from build123d import *
from build123d.topology import SkipClean

# Parameters (mm, degrees)
BOSS_EXTRUDE1_DEPTH   = 25
BOSS_EXTRUDE1_2_DEPTH = 25
BOSS_EXTRUDE1_3_DEPTH = 25
BOSS_EXTRUDE1_4_DEPTH = 25
BOSS_EXTRUDE1_5_DEPTH = 25
BOSS_EXTRUDE1_6_DEPTH = 25
BOSS_EXTRUDE1_7_DEPTH = 25
BOSS_EXTRUDE1_8_DEPTH = 25
BOSS_EXTRUDE2_START   = -3
SKETCH6_R             = 33
SKETCH6_R_2           = 31.685
BOSS_EXTRUDE2_DEPTH   = 3


with BuildPart() as part:
    # Sketch1 → Boss-Extrude1 (new body)
    with BuildSketch(Plane(origin=(0, 0, 0), x_dir=(-1, 0, 0), z_dir=(0, 0, 1))):
        with BuildLine():
            Line((-1.738225696, 20.20466707), (-2.272785403, 26.41824505))
            ThreePointArc((-2.272785403, 26.41824505), (-3.462351882, 28.561557475), (-5.853284272, 29.102204182))
            ThreePointArc((-5.853284272, 29.102204182), (-11.35995769, 27.425363923), (-16.439468924, 24.717262925))
            ThreePointArc((-16.439468924, 24.717262925), (-17.747818477, 22.644323466), (-17.073418251, 20.287622193))
            Line((-17.073418251, 20.287622193), (-13.05774592, 15.515968274))
            ThreePointArc((-13.05774592, 15.515968274), (-11.238150281, 14.485616628), (-9.187418979, 14.894338942))
            ThreePointArc((-9.187418979, 14.894338942), (-6.696960066, 16.167891819), (-4.035401805, 17.028374328))
            ThreePointArc((-4.035401805, 17.028374328), (-2.296305475, 18.189450019), (-1.738225696, 20.20466707))
        make_face()
    extrude(amount=BOSS_EXTRUDE1_DEPTH)



with BuildPart() as body_2:
    # Sketch1 → Boss-Extrude1 2 (new body)
    with BuildSketch(Plane(origin=(0, 0, 0), x_dir=(-1, 0, 0), z_dir=(0, 0, 1))):
        with BuildLine():
            Line((1.738225696, 20.20466707), (2.272785403, 26.41824505))
            ThreePointArc((2.272785403, 26.41824505), (3.462351882, 28.561557475), (5.853284272, 29.102204182))
            ThreePointArc((5.853284272, 29.102204182), (11.35995769, 27.425363923), (16.439468924, 24.717262925))
            ThreePointArc((16.439468924, 24.717262925), (17.747818477, 22.644323466), (17.073418251, 20.287622193))
            Line((17.073418251, 20.287622193), (13.05774592, 15.515968274))
            ThreePointArc((13.05774592, 15.515968274), (11.238150281, 14.485616628), (9.187418979, 14.894338942))
            ThreePointArc((9.187418979, 14.894338942), (6.696960066, 16.167891819), (4.035401805, 17.028374328))
            ThreePointArc((4.035401805, 17.028374328), (2.296305475, 18.189450019), (1.738225696, 20.20466707))
        make_face()
    extrude(amount=BOSS_EXTRUDE1_2_DEPTH)


with BuildPart() as body_3:
    # Sketch1 → Boss-Extrude1 3 (new body)
    with BuildSketch(Plane(origin=(0, 0, 0), x_dir=(-1, 0, 0), z_dir=(0, 0, 1))):
        with BuildLine():
            Line((15.515968274, 13.05774592), (20.287622193, 17.073418251))
            ThreePointArc((20.287622193, 17.073418251), (22.644323466, 17.747818477), (24.717262925, 16.439468924))
            ThreePointArc((24.717262925, 16.439468924), (27.425363923, 11.35995769), (29.102204182, 5.853284272))
            ThreePointArc((29.102204182, 5.853284272), (28.561557475, 3.462351882), (26.41824505, 2.272785403))
            Line((26.41824505, 2.272785403), (20.20466707, 1.738225696))
            ThreePointArc((20.20466707, 1.738225696), (18.189450019, 2.296305475), (17.028374328, 4.035401805))
            ThreePointArc((17.028374328, 4.035401805), (16.167891819, 6.696960066), (14.894338942, 9.187418979))
            ThreePointArc((14.894338942, 9.187418979), (14.485616628, 11.238150281), (15.515968274, 13.05774592))
        make_face()
    extrude(amount=BOSS_EXTRUDE1_3_DEPTH)


with BuildPart() as body_4:
    # Sketch1 → Boss-Extrude1 4 (new body)
    with BuildSketch(Plane(origin=(0, 0, 0), x_dir=(-1, 0, 0), z_dir=(0, 0, 1))):
        with BuildLine():
            Line((20.20466707, -1.738225696), (26.41824505, -2.272785403))
            ThreePointArc((26.41824505, -2.272785403), (28.561557475, -3.462351882), (29.102204182, -5.853284272))
            ThreePointArc((29.102204182, -5.853284272), (27.425363923, -11.35995769), (24.717262925, -16.439468924))
            ThreePointArc((24.717262925, -16.439468924), (22.644323466, -17.747818477), (20.287622193, -17.073418251))
            Line((20.287622193, -17.073418251), (15.515968274, -13.05774592))
            ThreePointArc((15.515968274, -13.05774592), (14.485616628, -11.238150281), (14.894338942, -9.187418979))
            ThreePointArc((14.894338942, -9.187418979), (16.167891819, -6.696960066), (17.028374328, -4.035401805))
            ThreePointArc((17.028374328, -4.035401805), (18.189450019, -2.296305475), (20.20466707, -1.738225696))
        make_face()
    extrude(amount=BOSS_EXTRUDE1_4_DEPTH)


with BuildPart() as body_5:
    # Sketch1 → Boss-Extrude1 5 (new body)
    with BuildSketch(Plane(origin=(0, 0, 0), x_dir=(-1, 0, 0), z_dir=(0, 0, 1))):
        with BuildLine():
            Line((13.05774592, -15.515968274), (17.073418251, -20.287622193))
            ThreePointArc((17.073418251, -20.287622193), (17.747818477, -22.644323466), (16.439468924, -24.717262925))
            ThreePointArc((16.439468924, -24.717262925), (11.35995769, -27.425363923), (5.853284272, -29.102204182))
            ThreePointArc((5.853284272, -29.102204182), (3.462351882, -28.561557475), (2.272785403, -26.41824505))
            Line((2.272785403, -26.41824505), (1.738225696, -20.20466707))
            ThreePointArc((1.738225696, -20.20466707), (2.296305475, -18.189450019), (4.035401805, -17.028374328))
            ThreePointArc((4.035401805, -17.028374328), (6.696960066, -16.167891819), (9.187418979, -14.894338942))
            ThreePointArc((9.187418979, -14.894338942), (11.238150281, -14.485616628), (13.05774592, -15.515968274))
        make_face()
    extrude(amount=BOSS_EXTRUDE1_5_DEPTH)


with BuildPart() as body_6:
    # Sketch1 → Boss-Extrude1 6 (new body)
    with BuildSketch(Plane(origin=(0, 0, 0), x_dir=(-1, 0, 0), z_dir=(0, 0, 1))):
        with BuildLine():
            Line((-1.738225696, -20.20466707), (-2.272785403, -26.41824505))
            ThreePointArc((-2.272785403, -26.41824505), (-3.462351882, -28.561557475), (-5.853284272, -29.102204182))
            ThreePointArc((-5.853284272, -29.102204182), (-11.35995769, -27.425363923), (-16.439468924, -24.717262925))
            ThreePointArc((-16.439468924, -24.717262925), (-17.747818477, -22.644323466), (-17.073418251, -20.287622193))
            Line((-17.073418251, -20.287622193), (-13.05774592, -15.515968274))
            ThreePointArc((-13.05774592, -15.515968274), (-11.238150281, -14.485616628), (-9.187418979, -14.894338942))
            ThreePointArc((-9.187418979, -14.894338942), (-6.696960066, -16.167891819), (-4.035401805, -17.028374328))
            ThreePointArc((-4.035401805, -17.028374328), (-2.296305475, -18.189450019), (-1.738225696, -20.20466707))
        make_face()
    extrude(amount=BOSS_EXTRUDE1_6_DEPTH)


with BuildPart() as body_7:
    # Sketch1 → Boss-Extrude1 7 (new body)
    with BuildSketch(Plane(origin=(0, 0, 0), x_dir=(-1, 0, 0), z_dir=(0, 0, 1))):
        with BuildLine():
            Line((-15.515968274, -13.05774592), (-20.287622193, -17.073418251))
            ThreePointArc((-20.287622193, -17.073418251), (-22.644323466, -17.747818477), (-24.717262925, -16.439468924))
            ThreePointArc((-24.717262925, -16.439468924), (-27.425363923, -11.35995769), (-29.102204182, -5.853284272))
            ThreePointArc((-29.102204182, -5.853284272), (-28.561557475, -3.462351882), (-26.41824505, -2.272785403))
            Line((-26.41824505, -2.272785403), (-20.20466707, -1.738225696))
            ThreePointArc((-20.20466707, -1.738225696), (-18.189450019, -2.296305475), (-17.028374328, -4.035401805))
            ThreePointArc((-17.028374328, -4.035401805), (-16.167891819, -6.696960066), (-14.894338942, -9.187418979))
            ThreePointArc((-14.894338942, -9.187418979), (-14.485616628, -11.238150281), (-15.515968274, -13.05774592))
        make_face()
    extrude(amount=BOSS_EXTRUDE1_7_DEPTH)


with BuildPart() as body_8:
    # Sketch1 → Boss-Extrude1 8 (new body)
    with BuildSketch(Plane(origin=(0, 0, 0), x_dir=(-1, 0, 0), z_dir=(0, 0, 1))):
        with BuildLine():
            Line((-20.20466707, 1.738225696), (-26.41824505, 2.272785403))
            ThreePointArc((-26.41824505, 2.272785403), (-28.561557475, 3.462351882), (-29.102204182, 5.853284272))
            ThreePointArc((-29.102204182, 5.853284272), (-27.425363923, 11.35995769), (-24.717262925, 16.439468924))
            ThreePointArc((-24.717262925, 16.439468924), (-22.644323466, 17.747818477), (-20.287622193, 17.073418251))
            Line((-20.287622193, 17.073418251), (-15.515968274, 13.05774592))
            ThreePointArc((-15.515968274, 13.05774592), (-14.485616628, 11.238150281), (-14.894338942, 9.187418979))
            ThreePointArc((-14.894338942, 9.187418979), (-16.167891819, 6.696960066), (-17.028374328, 4.035401805))
            ThreePointArc((-17.028374328, 4.035401805), (-18.189450019, 2.296305475), (-20.20466707, 1.738225696))
        make_face()
    extrude(amount=BOSS_EXTRUDE1_8_DEPTH)


with BuildPart() as part_1:
    with SkipClean():  # the faces are left unmerged after this step: merging them gives an invalid solid
        add(part.part)

        add(body_2.part)  # Revolve1 merges body 2

        add(body_3.part)  # Revolve1 merges body 3

        add(body_4.part)  # Revolve1 merges body 4

        add(body_5.part)  # Revolve1 merges body 5

        add(body_6.part)  # Revolve1 merges body 6

        add(body_7.part)  # Revolve1 merges body 7

        add(body_8.part)  # Revolve1 merges body 8
        # Sketch5 → Revolve1 (revolve)
        with BuildSketch(Plane(origin=(0, 0, 0), x_dir=(1, 0, 0), z_dir=(0, 1, 0))):
            with BuildLine():
                Line((17.5, -25), (31.685, -25))
                Line((31.685, -25), (31.685, -65))
                Line((31.685, -65), (0, -65))
                Line((0, -65), (0, -55.202941459))
                ThreePointArc((0, -55.202941459), (12.374368671, -50.07731013), (17.5, -37.702941459))
                Line((17.5, -37.702941459), (17.5, -25))
            make_face()
        revolve(axis=Axis((0, 0, 65), (0, 0, -1)))

    # Sketch6 → Boss-Extrude2 (add)
    with SkipClean():  # the faces are left unmerged after this step: merging them gives an invalid solid
        with BuildSketch(Plane(origin=(0, 0, 25), x_dir=(-1, 0, 0), z_dir=(0, 0, -1)).offset(BOSS_EXTRUDE2_START)):
            Circle(SKETCH6_R)
            with Locations(Location((0, 0, 0), (0, 0, 180))):
                Circle(SKETCH6_R_2, mode=Mode.SUBTRACT)
        extrude(amount=BOSS_EXTRUDE2_DEPTH)


solid = part_1.part
Source: CAD feature listing. Evaluate the final solid. Frame: model axes, mm. A direction names the side the tool comes from. Round coordinates to 2 decimals unless told otherwise and drop trailing zeros. Loops run counter-clockwise (first coordinate to the right, second up) from the corner with the lowest first, then second, coordinate; pieces in that order, holes last. Notation, with made-up numbers: (-4, -35) -> (18, -35) arc R19 cw to (18, -29) -> close; hole circle Ø11 at (64, 27.25). An arc over 180 degrees is marked (long way). Answer as a JSON object with one key per item and string values. Group by question number.
Q1. Section query C-C (z = 10.5). State how many separate pieces and enclosed holes the cut face has, plus the area to 3 significant figures.
Q2. Section query A-A (x = 0). Output: boundary loops of the cut face in (y, z) (3 decimals).
Q3. Access query for faces 4 (the cylindrical face through (17.743, -22.679, 12.325)), 5 (the cylindrical face through (27.394, 11.434, 12.325)), 6 (the cylindrical face through (30.22, -9.52, 46.76)), 7 (the flat face through (2, -23.27, 12.32)). Directions: +Z, -Z, +X, -X, +Y, -Y. A direction counts if a zero-diameter tool reaches every point of the face in a straight line with its end or side. Return the directions, or none.
Q4. Ray query, line 1 (Y direction, x = 0, z = 31) (3 decimals); line 2 (Z direction, x = -12, y = 30). Return the intervals inside material, ascending. Write a range as from..to.
Q5. Mould query, pull axis X, two halves, no side actions, for faces 1 (the cylindrical face through (28.54, -3.434, 12.325)), 2 (the flat face through (22, 10, 0)), 3 (the cylindrical face through (18.17, -2.31, 12.32)). Classes: pulls with the +X half, pulls with the -X half, needs draft (parallel to the pull), parting line crosses it, or undercut.
Q6. Contact query for flat-ended pins moving along their axis: P1, Ø1.5, axis at y = -10.5, z = 12, coming from the +X side; P2, Ø2, axis at y = -8.5, z = 46.5, coming from the +X side; P3, Ø1, axis at y = 25.5, z = 58.5, coming from the -X side; P4, Ø1, axis at x = -20, y = -15, coming from the -Z side. Output: stop coordinate, or through.
Q7. Section query D-D (x = -19). Output: boundary loops of the cut face in (y, z), plus the area to 3 significant figures.
Completed:
{
 "1": {"separate pieces": "8", "enclosed holes": "0", "area": "1,350 mm²"},
 "2": {"outline": "(-33, 25) -> (-17.5, 25) -> (-17.5, 37.703) arc R17.5 cw to (17.5, 37.703) -> (17.5, 25) -> (33, 25) -> (33, 28) -> (31.685, 28) -> (31.685, 65) -> (-31.685, 65) -> (-31.685, 28) -> (-33, 28) -> close"},
 "3": {"face 4": "-Z, +X", "face 5": "-Z, +X, +Y", "face 6": "+Z", "face 7": "-Z, -Y"},
 "4": {"line 1": "-31.685..-17.5, 17.5..31.685", "line 2": "25..28"},
 "5": {"face 1": "pulls with the +X half", "face 2": "needs draft", "face 3": "undercut"},
 "6": {"P1": "x = 28.04", "P2": "x = 30.78", "P3": "x = -19.47", "P4": "z = 0"},
 "7": {"outline": "(-26.98, 25) -> (-15.99, 25) -> (-15.99, 0) -> (-1.88, 0) -> (-1.88, 25) -> (1.88, 25) -> (1.88, 0) -> (15.99, 0) -> (15.99, 25) -> (26.98, 25) -> (26.98, 28) -> (25.36, 28) -> (25.36, 65) -> (-25.36, 65) -> (-25.36, 28) -> (-26.98, 28) -> close", "area": "2,740 mm²"}
}
